Geometry check sheet. Reference: the model listing, model coordinates, mm. A direction names the side the tool comes from. Give positions to 0.01 mm unless a question says otherwise; leave off trailing zeros. Loops run counter-clockwise (first coordinate to the right, second up) from the corner with the lowest first, then second, coordinate; pieces in that order, holes last. Notation, with made-up numbers: (-12.5, 86.5) -> (44.5, 86.5) arc R13 cw to (44.5, 102.5) -> close; hole circle Ø3 at (45, 8). An arc over 180 degrees is marked (long way). Write item = value, one per line.
```python
from build123d import *

# Parameters (mm, degrees)
ESBO_O1_W                 = 45
ESBO_O1_H                 = 26
RESSALTO_EXTRUS_O1_DEPTH  = 5
RESSALTO_EXTRUS_O4_START  = -5
ESBO_O6_W                 = 51
ESBO_O6_H                 = 32
ESBO_O6_W_2               = 45
ESBO_O6_H_2               = 26
RESSALTO_EXTRUS_O4_DEPTH  = 14
ESBO_O7_W                 = 49
ESBO_O7_H                 = 30
ESBO_O7_W_2               = 45
ESBO_O7_H_2               = 26
RESSALTO_EXTRUS_O5_DEPTH  = 50
ESBO_O8_W                 = 49
ESBO_O8_H                 = 30
RESSALTO_EXTRUS_O6_DEPTH  = 2
RESSALTO_EXTRUS_O9_DEPTH  = 15
ESBO_O11_R                = 5.5
RESSALTO_EXTRUS_O10_DEPTH = 35
ESBO_O9_W                 = 13
ESBO_O9_H                 = 19
CORTE_EXTRUS_O2_DEPTH     = 23
ESBO_O12_W                = 5
ESBO_O12_H                = 5
RESSALTO_EXTRUS_O11_DEPTH = 5
ESBO_O13_W                = 5
ESBO_O13_H                = 5
RESSALTO_EXTRUS_O12_DEPTH = 71
ESBO_O14_W                = 51
ESBO_O14_H                = 5
RESSALTO_EXTRUS_O13_DEPTH = 5
ESBO_O16_R                = 2
CORTE_EXTRUS_O4_DEPTH     = 3
ESBO_O17_R                = 1.5
CORTE_EXTRUS_O5_DEPTH     = 19
ESBO_O18_W                = 51
ESBO_O18_H                = 50
ESBO_O18_W_2              = 41
ESBO_O18_H_2              = 40
RESSALTO_EXTRUS_O14_DEPTH = 5
FILETE3_R                 = 5
ESBO_O19_W                = 51
ESBO_O19_H                = 1
CORTE_EXTRUS_O6_DEPTH     = 40


with BuildPart() as part:
    # Esboço1 → Ressalto-extrusão1 (new body)
    with BuildSketch(Plane.XY):
        Polygon((-25.5, 16), (-25.5, -16), (-22.5, -16), (22.5, -16), (25.5, -16), (25.5, 16), align=None)
        Rectangle(ESBO_O1_W, ESBO_O1_H, mode=Mode.SUBTRACT)
    extrude(amount=RESSALTO_EXTRUS_O1_DEPTH)

    # Esboço6 → Ressalto-extrusão4 (add)
    with BuildSketch(Plane(origin=(0, 0, 0), x_dir=(-1, 0, 0), z_dir=(0, 0, -1)).offset(RESSALTO_EXTRUS_O4_START)):
        Rectangle(ESBO_O6_W, ESBO_O6_H)
        Rectangle(ESBO_O6_W_2, ESBO_O6_H_2, mode=Mode.SUBTRACT)
    extrude(amount=-RESSALTO_EXTRUS_O4_DEPTH)

    # Esboço7 → Ressalto-extrusão5 (add)
    with BuildSketch(Plane.XY.offset(19)):
        Rectangle(ESBO_O7_W, ESBO_O7_H)
        Rectangle(ESBO_O7_W_2, ESBO_O7_H_2, mode=Mode.SUBTRACT)
    extrude(amount=RESSALTO_EXTRUS_O5_DEPTH)

    # Esboço8 → Ressalto-extrusão6 (add)
    with BuildSketch(Plane.XY.offset(69)):
        Rectangle(ESBO_O8_W, ESBO_O8_H)
    extrude(amount=RESSALTO_EXTRUS_O6_DEPTH)

    # Esboço10 → Ressalto-extrusão9 (add)
    with BuildSketch(Plane(origin=(0, 0, 69), x_dir=(-1, 0, 0), z_dir=(0, 0, -1))):
        with BuildLine():
            ThreePointArc((-2, 5.477225575), (-17, 0), (-2, -5.477225575))
            ThreePointArc((-2, -5.477225575), (13, 0), (-2, 5.477225575))
        make_face()
    extrude(amount=RESSALTO_EXTRUS_O9_DEPTH)

    # Esboço11 → Ressalto-extrusão10 (add)
    with BuildSketch(Plane(origin=(0, 0, 54), x_dir=(-1, 0, 0), z_dir=(0, 0, -1))):
        with BuildLine():
            ThreePointArc((-2, -5.477225575), (13, 0), (-2, 5.477225575))
            ThreePointArc((-2, 5.477225575), (-17, 0), (-2, -5.477225575))
        make_face()
        with Locations((-8.5, 0)):
            Circle(ESBO_O11_R, mode=Mode.SUBTRACT)
        with Locations((4.5, 0)):
            Circle(ESBO_O11_R, mode=Mode.SUBTRACT)
    extrude(amount=RESSALTO_EXTRUS_O10_DEPTH)

    # Esboço9 → Corte-extrusão2 (cut)
    with BuildSketch(Plane(origin=(0, 15, 0), x_dir=(1, 0, 0), z_dir=(0, 1, 0))):
        with Locations((-16, -59.5)):
            Rectangle(ESBO_O9_W, ESBO_O9_H)
    extrude(amount=-CORTE_EXTRUS_O2_DEPTH, mode=Mode.SUBTRACT)

    # Esboço12 → Ressalto-extrusão11 (add)
    with BuildSketch(Plane.XY):
        with Locations((23, -18.5)):
            Rectangle(ESBO_O12_W, ESBO_O12_H)
        with Locations((-23, -18.5)):
            Rectangle(ESBO_O12_W, ESBO_O12_H)
    extrude(amount=RESSALTO_EXTRUS_O11_DEPTH)

    # Esboço13 → Ressalto-extrusão12 (add)
    with BuildSketch(Plane(origin=(0, 0, 0), x_dir=(-1, 0, 0), z_dir=(0, 0, -1))):
        with Locations((23, -23.5)):
            Rectangle(ESBO_O13_W, ESBO_O13_H)
        with Locations((-23, -23.5)):
            Rectangle(ESBO_O13_W, ESBO_O13_H)
    extrude(amount=-RESSALTO_EXTRUS_O12_DEPTH)

    # Esboço14 → Ressalto-extrusão13 (add)
    with BuildSketch(Plane.XY.offset(71)):
        with Locations((0, -23.5)):
            Rectangle(ESBO_O14_W, ESBO_O14_H)
    extrude(amount=-RESSALTO_EXTRUS_O13_DEPTH)

    # Esboço16 → Corte-extrusão4 (cut)
    with BuildSketch(Plane.ZY.offset(24.5)):
        with Locations((29, -11)):
            Circle(ESBO_O16_R)
    extrude(amount=-CORTE_EXTRUS_O4_DEPTH, mode=Mode.SUBTRACT)

    # Esboço17 → Corte-extrusão5 (cut, symmetric)
    with BuildSketch(Plane(origin=(0, 0, 0), x_dir=(0, 0, -1), z_dir=(1, 0, 0))):
        with Locations((-52.5, 0)):
            Circle(ESBO_O17_R)
    extrude(amount=CORTE_EXTRUS_O5_DEPTH, both=True, mode=Mode.SUBTRACT)

    # Esboço18 → Ressalto-extrusão14 (add)
    with BuildSketch(Plane.XY.offset(71)):
        with Locations((0, -46)):
            Rectangle(ESBO_O18_W, ESBO_O18_H)
        with Locations((0, -46)):
            Rectangle(ESBO_O18_W_2, ESBO_O18_H_2, mode=Mode.SUBTRACT)
    extrude(amount=-RESSALTO_EXTRUS_O14_DEPTH)

    # Filete3
    # the kernel refuses this fillet: 5 mm, written as the material it adds along each edge
    with BuildSketch(Plane(origin=(20.5, -21, 5), x_dir=(0, 1, 0), z_dir=(1, 0, 0)), Plane(origin=(-20.5, -21, 5), x_dir=(0, 0, 1), z_dir=(-1, 0, 0)), Plane(origin=(25.5, -26, 66), x_dir=(0, 0, -1), z_dir=(-1, 0, 0)), Plane(origin=(-20.5, -26, 66), x_dir=(0, 0, -1), z_dir=(-1, 0, 0))) as filete3_piece_1:
        with BuildLine():
            CenterArc((FILETE3_R, FILETE3_R), FILETE3_R, 180, 90)
            Line((0, FILETE3_R), (0, 0))
            Line((0, 0), (FILETE3_R, 0))
        make_face()
    extrude(amount=5)
    # the kernel refuses this fillet: 5 mm, written as the material it takes off along each edge
    with BuildSketch(Plane(origin=(-38, -26, 0), x_dir=(0, 0, 1), z_dir=(1, 0, 0))) as filete3_2_piece_1:
        with BuildLine():
            CenterArc((FILETE3_R, -FILETE3_R), FILETE3_R, 90, 90)
            Line((0, -FILETE3_R), (0, 0))
            Line((0, 0), (FILETE3_R, 0))
        make_face()
    extrude(amount=30, mode=Mode.SUBTRACT)
    with BuildSketch(Plane(origin=(8, -26, 0), x_dir=(0, 1, 0), z_dir=(1, 0, 0))) as filete3_2_piece_2:
        with BuildLine():
            CenterArc((FILETE3_R, FILETE3_R), FILETE3_R, 180, 90)
            Line((0, FILETE3_R), (0, 0))
            Line((0, 0), (FILETE3_R, 0))
        make_face()
    extrude(amount=30, mode=Mode.SUBTRACT)

    # Esboço19 → Corte-extrusão6 (cut)
    with BuildSketch(Plane.XZ.offset(71)):
        with Locations((0, 68.5)):
            Rectangle(ESBO_O19_W, ESBO_O19_H)
    extrude(amount=-CORTE_EXTRUS_O6_DEPTH, mode=Mode.SUBTRACT)


solid = part.part
```
Item 1: Tool access check on faces 1 (the flat face through (23, -26, 33)), 2 (the flat face through (22.5, 0, 34)), 3 (the flat face through (-10, 1, 69)). Record the directions out of +Z, -Z, +X, -X, +Y, -Y that give a thin tool (end or side, any length) a straight path to the whole face; none if there is none.
Answer:
face_1 = -Z, +X, -X, -Y
face_2 = -Z
face_3 = none
Item 2: Section check A-A, the plane y = -11. Record the cut outline in (x, z), plus the area to 3 significant figures.
Answer:
outline = (-25.5, 0) -> (-22.5, 0) -> (-22.5, 27) -> (-24.5, 27) -> (-24.5, 19) -> (-25.5, 19) -> close; (-24.5, 31) -> (-22.5, 31) -> (-22.5, 69) -> (22.5, 69) -> (22.5, 0) -> (25.5, 0) -> (25.5, 19) -> (24.5, 19) -> (24.5, 71) -> (-24.5, 71) -> close
area = 404 mm^2
Item 3: Gauge pin test, flat ends, axial feed: pin 1 (2.5 mm diameter, centred on x = 23, z = 23.5, fed in from -Y); pin 2 (8 mm diameter, centred on y = -5, z = 46, fed in from -X); pin 3 (0.8 mm diameter, centred on x = 22.5, z = 68.5, fed in from -Y). Record the tip position at first contact, or that the pin passes through.
Answer:
pin_1 = -26
pin_2 = -24.5
pin_3 = -31
Item 4: Thickness scan on L1, parallel to Y at x = -4.5, z = 32; L2, parallel to X at y = 0, z = 43; L3, parallel to X at y = -12.5, z = 47.5. Record the ranges inside material, lowest first. Write a range as [from, to].
Answer:
L1 = [-15, -13], [-8.5, -5.5], [5.5, 8.5], [13, 15]
L2 = [-24.5, -22.5], [-13, -10], [1, 3], [14, 17], [22.5, 24.5]
L3 = [-24.5, -22.5], [22.5, 24.5]
Item 5: Section check D-D, the plane x = -16. Record the cut outline in (y, z).
Answer:
outline = (-71, 66) -> (-66, 66) -> (-66, 68) -> (-71, 68) -> close; (-71, 69) -> (-66, 69) -> (-66, 71) -> (-71, 71) -> close; (-26, 66) -> (-21, 66) -> (-21, 71) -> (-26, 71) -> close; (-16, 0) -> (-13, 0) -> (-13, 69) -> (15, 69) -> (15, 71) -> (-15, 71) -> (-15, 19) -> (-16, 19) -> close; (13, 0) -> (16, 0) -> (16, 19) -> (15, 19) -> (15, 50) -> (13, 50) -> close
Item 6: Section check C-C, the plane x = 8.5. Give the number of separate pieces and of enclosed holes in the cut face, plus the area to 3 significant figures.
Answer:
separate_pieces = 4
enclosed_holes = 0
area = 884 mm^2
Item 7: Section check B-B, the plane z = 43.5. Record the cut outline in (x, y), plus the area to 3 significant figures.
Answer:
outline = (-25.5, -26) -> (-20.5, -26) -> (-20.5, -21) -> (-25.5, -21) -> close; (-24.5, -15) -> (24.5, -15) -> (24.5, 15) -> (-24.5, 15) -> close; (2, -5.48) arc R8.5 ccw (long way) to (2, 5.48) arc R8.5 ccw (long way) to start; (20.5, -26) -> (25.5, -26) -> (25.5, -21) -> (20.5, -21) -> close; hole (-22.5, -13) -> (22.5, -13) -> (22.5, 13) -> (-22.5, 13) -> close; hole circle Ø11 at (-4.5, 0); hole circle Ø11 at (8.5, 0)
area = 584 mm^2
Item 8: Draft check along Z on faces 4 (the flat face through (-2, -67, 68)), 5 (the cylindrical face through (23, -25, 2)), 6 (the flat face through (-9.5, 14, 60)), 7 (the flat face through (-25.5, -21.3, 27.8)). Enter one of: +Z half, -Z half, draft (parallel to the pull), parting line (faces both ways), or undercut.
Answer:
face_4 = undercut
face_5 = -Z half
face_6 = undercut
face_7 = draft
